```python
from build123d import *

# Parameters (mm, degrees)
EXTRUDE1_DEPTH = 10
EXTRUDE2_DEPTH = 5
DRAFT1_ANGLE   = 10


with BuildPart() as part:
    # Sketch1 → Extrude1 (new body)
    with BuildSketch(Plane.XY):
        with BuildLine():
            Line((0, 15), (0, -15))
            ThreePointArc((0, -15), (15, 0), (0, 15))
        make_face()
    extrude(amount=EXTRUDE1_DEPTH)

    # Sketch2 → Extrude2 (add)
    with BuildSketch(Plane(origin=(0, 0, 0), x_dir=(0, 0, -1), z_dir=(1, 0, 0))):
        Polygon((-10, 18), (-10, -18), (-18.164261824, -12.225501851), (-23.803781668, 12.130109739), align=None)
    extrude(amount=EXTRUDE2_DEPTH)

    # Draft1
    draft1_faces = [part.faces().sort_by_distance(p)[0] for p in [
        (2.5, -15.112750925, 14.082130912),
        (2.5, -0.047696056, 20.984021746),
        (2.5, 15.06505487, 16.901890834),
    ]]
    draft(draft1_faces, Plane(origin=(0, 0, 0), x_dir=(0, 0, 1), z_dir=(1, 0, 0)), DRAFT1_ANGLE)


solid = part.part
```
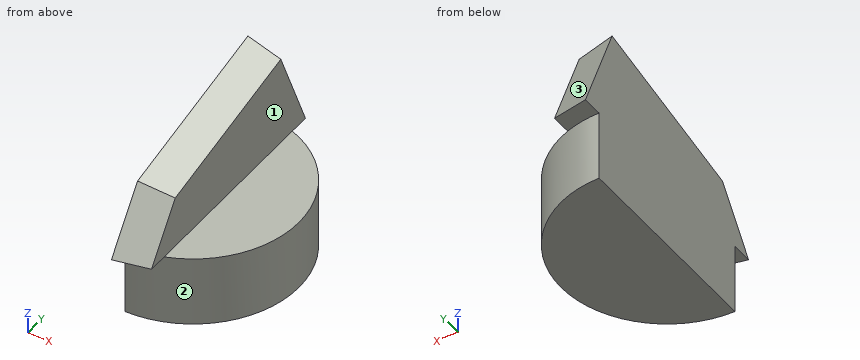
Model file for the job. Use its own axes, mm. Face numbers are marked on the shaded views. A direction names the side the tool comes from. Coordinates: 2 decimals unless noted, no trailing zeros. Loops run counter-clockwise (first coordinate to the right, second up) from the corner with the lowest first, then second, coordinate; pieces in that order, holes last. Notation, with made-up numbers: (49.5, 71.25) - (78.5, 71.25) arc R21 ccw to (78.5, 101.25) - close; hole circle Ø6 at (51.5, 18). An arc over 180 degrees is marked (long way). Answer as a JSON object with one key per item and string values. Group by question number.
(1) Cut at B-B (x = 1.25). Give the cut face in (y, z), then the cut area to 3 significant figures.
(2) Probe line 1 along X through (y, z) = (-9.5, 11.5); line 2 along X through (y, z) = (0, 4.5); line 3 along Z through (x, y) = (9.5, 3). List the from-to ranges inside material, lowest first.
(3) Cut at A-A (y = 7). Give the cut face in (x, z).
(4) Cut at D-D (y = -7). Give the cut face in (x, z), then the cut area to 3 significant figures.
(5) Cut at C-C (z = 2). Give the cut face in (x, y).
(6) Flat gauge pins, fed straight in: pin 1 (6.5 mm diameter, centred on y = -7.5, z = 14, fed in from +X); pin 2 (1.5 mm diameter, centred on x = 7.5, z = 9, fed in from +Y); pin 3 (3 mm diameter, centred on x = 9, y = 6.5, fed in from +Z). Where does each tip first touch, or does it go through?
(7) Tool access for the marked faces 1, 2 and 3: list every direction of +Z, -Z, +X, -X, +Y, -Y with a clear straight run to the whole face (end or side of a thin tool).
Geometry says:
{
 "1": {"outline": "(-17.73, 10) - (-14.95, 10) - (-14.95, 0) - (14.95, 0) - (14.95, 10) - (17.76, 10) - (12, 23.55) - (-12.09, 17.97) - close", "area": "620 mm^2"},
 "2": {"line 1": "x = 0 to 5", "line 2": "x = 0 to 15", "line 3": "z = 0 to 10"},
 "3": {"outline": "(0, 0) - (13.27, 0) - (13.27, 10) - (5, 10) - (5, 21.71) - (0, 22.62) - close"},
 "4": {"outline": "(0, 0) - (13.27, 0) - (13.27, 10) - (5, 10) - (5, 18.47) - (0, 19.37) - close", "area": "177 mm^2"},
 "5": {"outline": "(0, -15) arc R15 ccw to (0, 15) - close"},
 "6": {"pin 1": "stops at x = 5", "pin 2": "stops at y = 13.4", "pin 3": "stops at z = 10"},
 "7": {"face 1": "+Z, +X, +Y, -Y", "face 2": "-Z, +X", "face 3": "+Z, +X, +Y"}
}
